Input: dimensioned drawing with shaded views. Units: mm. Origin: part minimum x, y, z. Round coordinates to 2 decimals unless told otherwise and drop trailing zeros. Loops run counter-clockwise (first coordinate to the right, second up) from the corner with the lowest first, then second, coordinate; pieces in that order, holes last. Notation, with made-up numbers: (-0.75, 13.5) - (11.25, 13.5) arc R21 ccw to (11.25, 19.5) - close; hole circle Ø4 at (15, 60). An arc over 180 degrees is marked (long way). One line per question, with ' | ' between items. Start each with the question number.
1. Cut plane A-A (x = 93.8). Return loops of the section in (y, z).
2. Cut plane C-C (y = 18). Return loops of the section in (x, z), then the cut area to 3 significant figures.
3. Cut plane D-D (x = 74). Return loops of the section in (y, z).
4. Ray query, line 1 (Y direction, x = 7.8, z = 3.25); line 2 (Y direction, x = 67, z = 5.5); line 3 (Y direction, x = 48, z = 3.5). Return the intervals inside material, ascending.
5. Pin query (flat end, axial travel): pin 1 (3 mm diameter, centred on y = 62, z = 3, fed in from +X); pin 2 (1.9 mm diameter, centred on y = 61.5, z = 4.5, fed in from -X); pin 3 (3 mm diameter, centred on x = 47.5, z = 3, fed in from +Y). Return the tip coordinate at first contact, or that it passes through.
6. Cut plane B-B (z = 4.5). Return loops of the section in (x, y) (1 decimal), then the cut area to 3 significant figures.
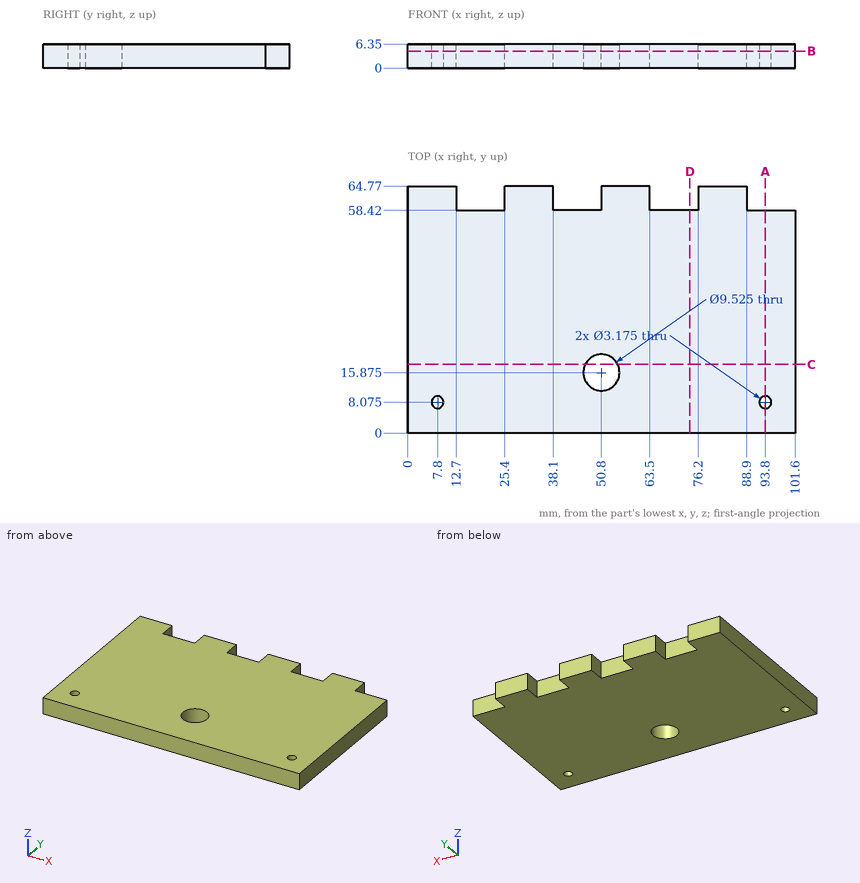
Answers follow:
1) outline: (0, 0) - (6.49, 0) - (6.49, 6.35) - (0, 6.35) - close; (9.66, 0) - (58.42, 0) - (58.42, 6.35) - (9.66, 6.35) - close
2) outline: (0, 0) - (46.54, 0) - (46.54, 6.35) - (0, 6.35) - close; (55.06, 0) - (101.6, 0) - (101.6, 6.35) - (55.06, 6.35) - close | area: 591 mm2
3) outline: (0, 0) - (58.42, 0) - (58.42, 6.35) - (0, 6.35) - close
4) line 1: y = 0 to 6.49, 9.66 to 64.77 | line 2: y = 0 to 58.42 | line 3: y = 0 to 12.02, 19.73 to 58.42
5) pin 1: stops at x = 88.9 | pin 2: stops at x = 0 | pin 3: stops at y = 58.42
6) outline: (0, 0) - (101.6, 0) - (101.6, 58.4) - (88.9, 58.4) - (88.9, 64.8) - (76.2, 64.8) - (76.2, 58.4) - (63.5, 58.4) - (63.5, 64.8) - (50.8, 64.8) - (50.8, 58.4) - (38.1, 58.4) - (38.1, 64.8) - (25.4, 64.8) - (25.4, 58.4) - (12.7, 58.4) - (12.7, 64.8) - (0, 64.8) - close; hole circle Ø3.2 at (7.8, 8.1); hole circle Ø9.5 at (50.8, 15.9); hole circle Ø3.2 at (93.8, 8.1) | area: 6,170 mm2
